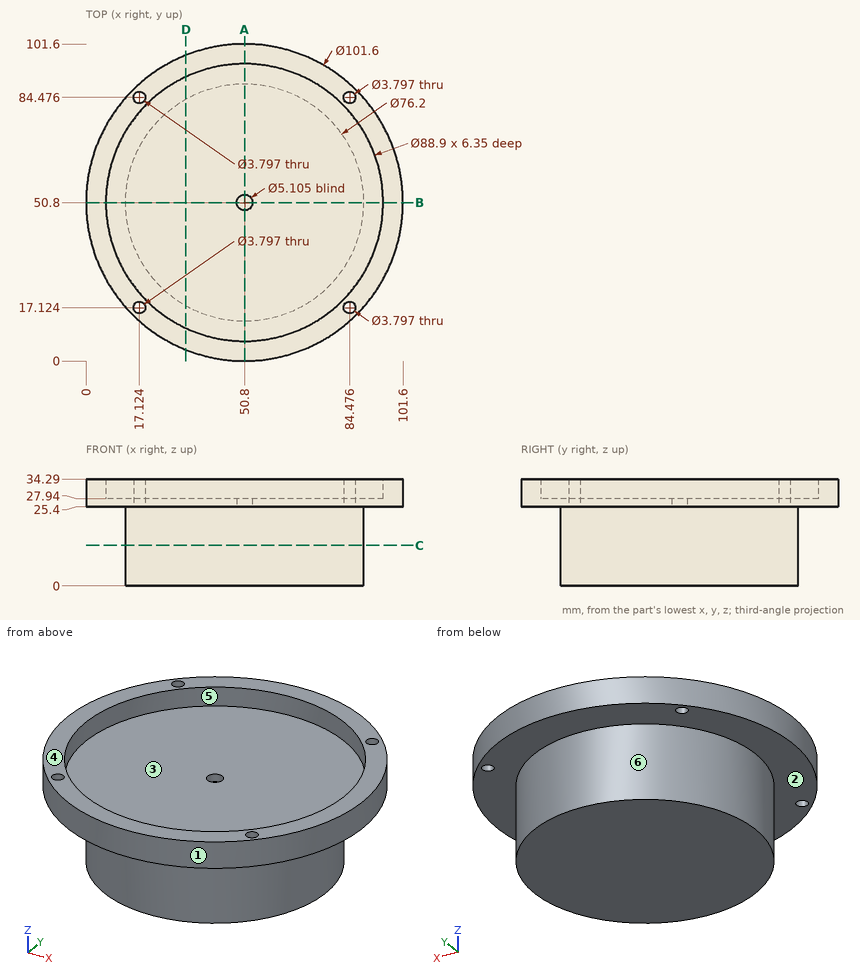
For this review, use the dimensioned drawing (mm, ordinates from the lowest corner) and the shaded views. A direction names the side the tool comes from. Coordinates: 2 decimals unless noted, no trailing zeros. Order: outer loops, then holes, each group sorted by start corner. A loop starts at its lowest first (then second) coordinate and runs counter-clockwise, first axis right, second up. Notation, with made-up numbers: (33, -2.75) - (68, -2.75) arc R32 cw to (68, 33.25) - close; hole circle Ø11 at (69, -27.75). An arc over 180 degrees is marked (long way). Answer as a JSON object with one key per item and string values. Group by question number.
1. We need section A-A on x = 50.8. State the section outline as (y, z) points.
2. We need section D-D on x = 32. State the section outline as (y, z) points, then the cut area to 3 significant figures.
3. For probe 1 along X at (y, z) = (50, 32); probe 2 along Z at (x, y) = (18.5, 39); probe 3 along Z at (x, y) = (77.5, 84), list the stretches that pass through material, from the lowest coordinate up.
4. Clearance check with flat-ended pins moving along their axes: P1, Ø1.5, axis at x = 30, z = 9.5, coming from the +Y side; P2, Ø4, axis at x = 51.5, y = 21.5, coming from the +Z side; P3, Ø5, axis at x = 61.5, z = 7, coming from the -Y side; P4, Ø2.5, axis at x = 84.48, y = 17.12, coming from the -Z side. State where each tip first meets the part, or that it passes through.
5. We need section C-C on z = 13. State the section outline as (x, y) points, then the cut area to 3 significant figures.
6. For the marked faces 1, 2 and 3, list the 3-axis set-ups (+Z, -Z, +X, -X, +Y, -Y) from which the entire face can be reached by the end or side of a thin tool; tool diameter is ignored.
7. The part is to be moulded in two halves that separate along Y. For the marked faces 4, 5 and 6, say which applies: pulls with the +Y half, pulls with the -Y half, needs draft (parallel to the pull), parting line crosses it, or undercut.
Final values:
{
 "1": {"outline": "(0, 25.4) - (12.7, 25.4) - (12.7, 0) - (88.9, 0) - (88.9, 25.4) - (101.6, 25.4) - (101.6, 34.29) - (95.25, 34.29) - (95.25, 27.94) - (53.35, 27.94) - (53.35, 25.4) - (48.25, 25.4) - (48.25, 27.94) - (6.35, 27.94) - (6.35, 34.29) - (0, 34.29) - close"},
 "2": {"outline": "(3.61, 25.4) - (17.66, 25.4) - (17.66, 0) - (83.94, 0) - (83.94, 25.4) - (97.99, 25.4) - (97.99, 34.29) - (91.08, 34.29) - (91.08, 27.94) - (10.52, 27.94) - (10.52, 34.29) - (3.61, 34.29) - close", "area": "2,010 mm²"},
 "3": {"probe 1": "0.01 to 6.36, 95.24 to 101.59", "probe 2": "0 to 27.94", "probe 3": "25.4 to 27.94"},
 "4": {"P1": "y = 83.2", "P2": "z = 27.94", "P3": "y = 13.59", "P4": "through"},
 "5": {"outline": "circle Ø76.2 at (50.8, 50.8)", "area": "4,560 mm²"},
 "6": {"face 1": "+Z, -Z", "face 2": "-Z", "face 3": "+Z"},
 "7": {"face 4": "needs draft", "face 5": "undercut", "face 6": "parting line crosses it"}
}
